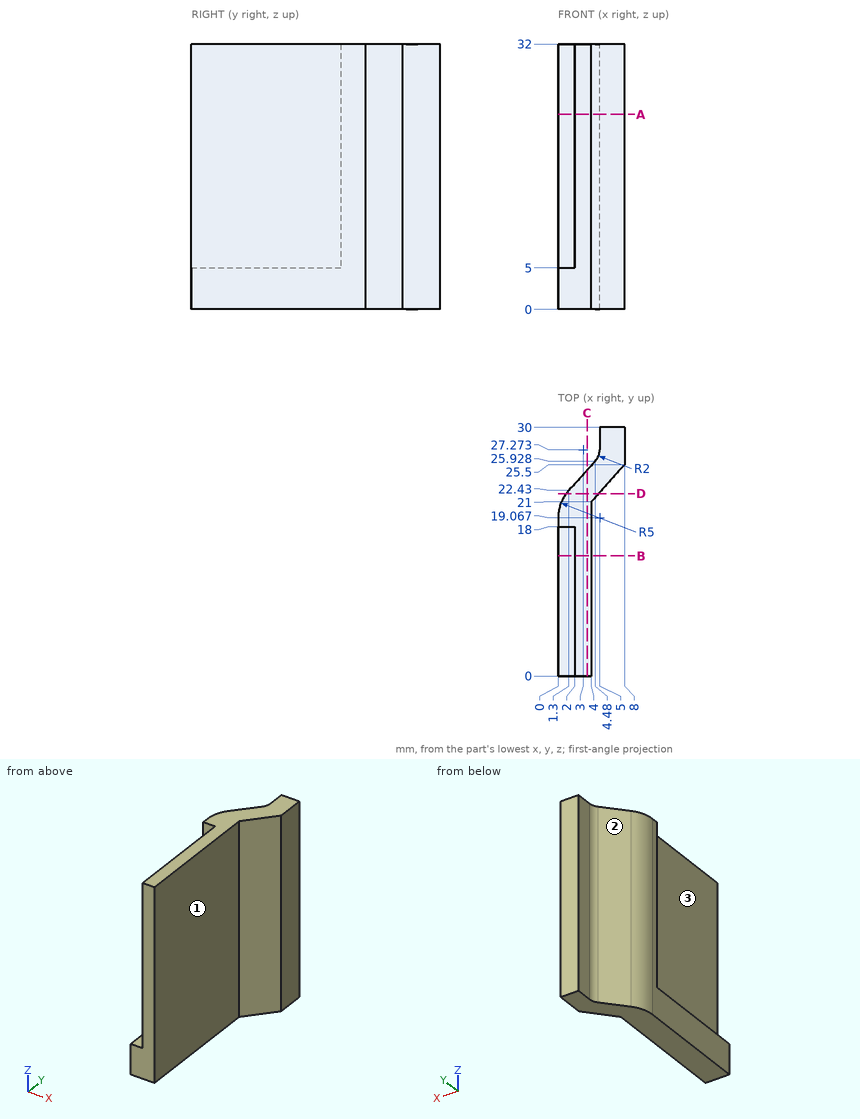
Can you work these out from the drawing? Everything is in mm from the part's minimum corner. A direction names the side the tool comes from. Round coordinates to 2 decimals unless told otherwise and drop trailing zeros. Loops run counter-clockwise (first coordinate to the right, second up) from the corner with the lowest first, then second, coordinate; pieces in that order, holes last. Notation, with made-up numbers: (-25.5, 31) - (-15.5, 31) arc R8 cw to (-15.5, 40) - close; hole circle Ø5 at (4.25, 64.25). An arc over 180 degrees is marked (long way). Write item = value, one per line. Start each with the question number.
(1) For P1, Ø0.6, axis at x = 1, y = 7, coming from the +Z side; P2, Ø0.6, axis at x = 1, z = 23.5, coming from the -Y side; P3, Ø1.5, axis at x = 6, z = 10, coming from the -Y side (1 decimal), each with a flat end and sliding along its axis, tell me the tip position at first contact or that it passes through.
(2) If we section it at B-B (y = 14.5): Please give me the cut outline in (x, z), and give its area (3 significant figures).
(3) If we section it at C-C (x = 3.5): Please give me the cut outline in (y, z).
(4) For the marked faces 1, 2 and 3, which set-ups out of +Z, -Z, +X, -X, +Y, -Y let a thin tool reach every point of the face, with its end or its side?
(5) If we section it at D-D (y = 22): Please give me the cut outline in (x, z), and give its area (3 significant figures).
(6) If we section it at A-A (z = 23.5): Please give me the cut outline in (x, y).
(7) If I drill on probe 1 along X at (y, z) = (4.5, 24); probe 2 along Z at (x, y) = (1.5, 12.5); probe 3 along Y at (x, z) = (6.75, 5) (1 decimal), over which ranges is the centre line in solid material (lowest first)? Write a range as [from, to].
Ans:
q1.P1 = 5
q1.P2 = 18
q1.P3 = 22.4
q2.outline = (0, 0) - (4, 0) - (4, 32) - (2, 32) - (2, 5) - (0, 5) - close
q2.area = 74.0 mm²
q3.outline = (0, 0) - (24.85, 0) - (24.85, 32) - (0, 32) - close
q4.face_1 = +Z, -Z, +X, -Y
q4.face_2 = +Z, -Z, -X, +Y
q4.face_3 = +Z, -X, -Y
q5.outline = (0.95, 0) - (4.89, 0) - (4.89, 32) - (0.95, 32) - close
q5.area = 126 mm²
q6.outline = (0, 18) - (2, 18) - (2, 0) - (4, 0) - (4, 21) - (8, 25.5) - (8, 30) - (5, 30) - (5, 27.27) arc R2 cw to (4.48, 25.93) - (1.3, 22.43) arc R5 ccw to (0, 19.07) - close
q7.probe_1 = [2, 4]
q7.probe_2 = [0, 5]
q7.probe_3 = [24.1, 30]
